Could you check a few things on this drawing? It's one solid part, dimensions in mm from its lowest x, y, z. A direction names the side the tool comes from. Coordinates: 2 decimals unless noted, no trailing zeros. Write each loop counter-clockwise with the first axis right and the second up, starting at its lowest first coordinate (ties: lowest second). Pieces come first, ordered by that corner, then holes.
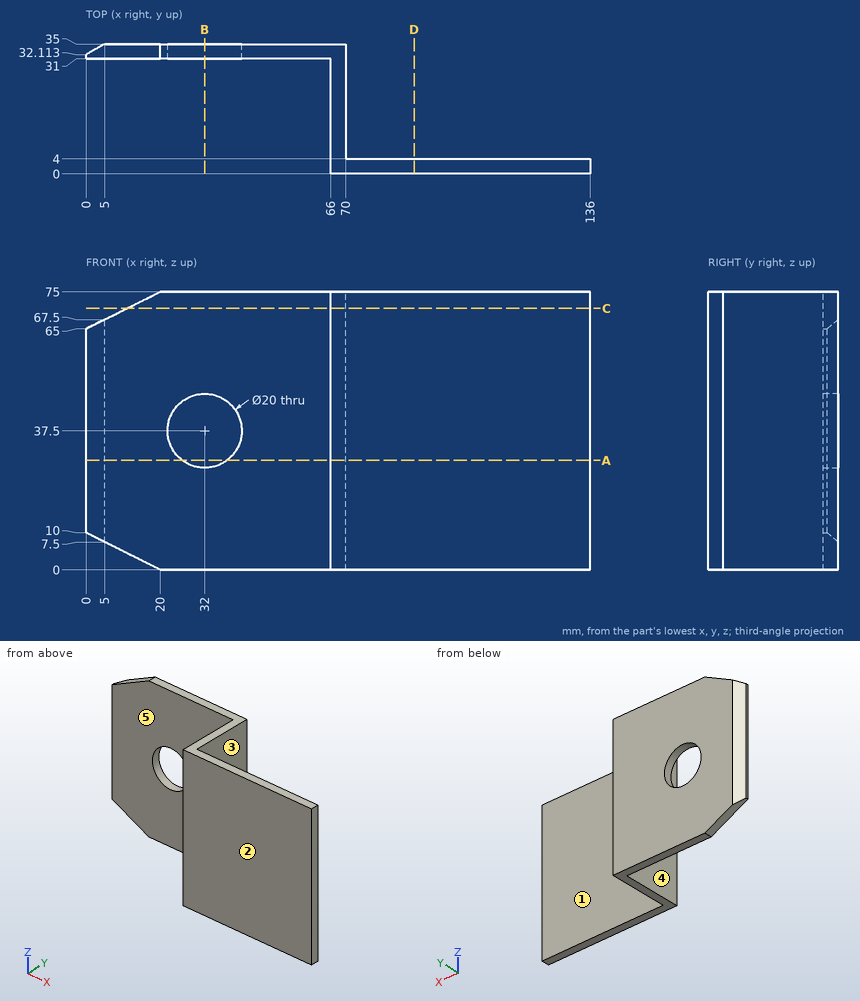
1) Imagine slicing it at B-B on x = 32. Please give me the cut outline in (y, z).
Values follow:
outline: (31, 0) - (35, 0) - (35, 27.5) - (31, 27.5) - close; (31, 47.5) - (35, 47.5) - (35, 75) - (31, 75) - close
2) Imagine slicing it at D-D on x = 88.5. Please give me the cut outline in (y, z).
Values follow:
outline: (0, 0) - (4, 0) - (4, 75) - (0, 75) - close
3) Will these pins go through, and if not, where does the flat tip stop? pin 1 (16 mm diameter, centred on x = 32, z = 37.5, fed in from -Y); pin 2 (9.5 mm diameter, centred on y = 22.5, z = 25, fed in from -X); pin 3 (9.5 mm diameter, centred on y = 16.5, z = 23, fed in from +X); pin 4 (20 mm diameter, centred on x = 27.5, z = 48, fed in from -Y).
Values follow:
pin 1: passes through
pin 2: stops at x = 66
pin 3: stops at x = 70
pin 4: stops at y = 31
4) Imagine slicing it at C-C on z = 70.5. Please give me the cut outline in (x, y).
Values follow:
outline: (11, 31) - (66, 31) - (66, 0) - (136, 0) - (136, 4) - (70, 4) - (70, 35) - (11, 35) - close
5) I need wall thicknesses on probe 1 along X at (y, z) = (32, 37); probe 2 along X at (y, z) = (2, 14); probe 3 along Y at (x, z) = (114, 8). Which ranges of each line are inside material? Lowest first, please.
Values follow:
probe 1: x = 0 to 22.01, 41.99 to 70
probe 2: x = 66 to 136
probe 3: y = 0 to 4
6) On a 3-axis mill with a long thin cutter (end or side, diameter ignored), from which of +Z, -Z, +X, -X, +Y, -Y can I reach the whole of each face in a straight line? I mean the marked faces 1 and 2. Say none if no direction works.
Values follow:
face 1: +Z, -Z, +X, +Y
face 2: +Z, -Z, +X, -X, -Y
7) We'd pull the mould along X, two halves only. Please class the marked faces 3, 4 and 5: pulls with the +X half, pulls with the -X half, needs draft (parallel to the pull), parting line crosses it, or undercut.
Values follow:
face 3: pulls with the +X half
face 4: pulls with the -X half
face 5: needs draft
8) Imagine slicing it at A-A on z = 29.5. Please give me the cut outline in (x, y).
Values follow:
outline: (0, 31) - (26, 31) - (26, 35) - (5, 35) - (0, 32.11) - close; (38, 31) - (66, 31) - (66, 0) - (136, 0) - (136, 4) - (70, 4) - (70, 35) - (38, 35) - close
